Source: CAD feature listing. Evaluate the final solid. Frame: model axes, mm. A direction names the side the tool comes from. Give positions to 0.01 mm unless a question says otherwise; leave off trailing zeros. Write each loop counter-clockwise with the first axis right and the second up, starting at its lowest first coordinate (ties: lowest second). Pieces come first, ordered by that corner, then holes.
```python
from build123d import *

# Parameters (mm, degrees)
F1_DEPTH      = 50.8
F3_DEPTH      = 49.1127015481
F3_DEPTH_BACK = 66.494050136
F4_R          = 5.0698297576
F4_W          = 24.7860401869
F4_H          = 10.0980177522
F5_DEPTH      = 86.2099544535
F5_DEPTH_BACK = 86.2099544535


with BuildPart() as f1:
    # F0 (on Top) → F1 (new body)
    with BuildSketch(Plane.XY):
        Polygon((-86.2089544535, 49.1117015481), (-86.2089544535, -49.1117015481), (-12.8575693816, -49.1117015481), (-12.8575693816, -66.493050136), (9.0635353699, -66.493050136), (9.0635353699, -49.1117015481), (86.2089544535, -49.1117015481), (86.2089544535, 49.1117015481), align=None)
    extrude(amount=F1_DEPTH)

    # F2 (on Front) → F3 (cut, two sides)
    with BuildSketch(Plane.XZ) as f3_sk:
        Polygon((9.0635353699, 50.8), (-12.8575693816, 50.8), (86.2089544535, 0), (86.2089544535, 50.8), align=None)
    extrude(amount=-F3_DEPTH, mode=Mode.SUBTRACT)
    extrude(f3_sk.sketch, amount=F3_DEPTH_BACK, mode=Mode.SUBTRACT)

    # F4 (on Right) → F5 (cut, two sides)
    with BuildSketch(Plane.YZ) as f5_sk:
        with Locations((-29.1465427727, 37.8675609827)):
            Circle(F4_R)
        with Locations((-29.1465427727, 14.9175236002)):
            Circle(F4_R)
        with Locations((20.425543189, 14.9175236002)):
            Circle(F4_R)
        with Locations((20.425543189, 37.8675609827)):
            Circle(F4_R)
        with Locations((-8.0325044692, 45.7509911239)):
            Rectangle(F4_W, F4_H)
    extrude(amount=-F5_DEPTH, mode=Mode.SUBTRACT)
    extrude(f5_sk.sketch, amount=F5_DEPTH_BACK, mode=Mode.SUBTRACT)


solid = f1.part
```
1. Access query for faces 5 (the cylindrical face through (-8.53, 19.327, 9.968)), 6 (the flat face through (-12.858, -58, 25)), 7 (the flat face through (39, -49.112, 15)), 8 (the flat face through (-39, -20.426, 46)), 9 (the flat face through (-50, -35, 50.8)). Directions: +Z, -Z, +X, -X, +Y, -Y. A direction counts if a zero-diameter tool reaches every point of the face in a straight line with its end or side. Return the directions, or none.
2. Cut plane C-C, the plane y = -9. Return the cut outline in (x, z), then the cut area to 3 significant figures.
3. Cut plane B-B, the plane x = -16. Return the cut outline in (y, z), then the cut area to 3 significant figures.
4. Contact query for flat-ended pins moving along their axis: P1, Ø3, axis at x = -52, z = 45, coming from the -Y side; P2, Ø8.5, axis at y = -55, z = 33, coming from the -X side; P3, Ø4, axis at x = 61.5, z = 14, coming from the +Y side; P4, Ø12.5, axis at x = -38.5, y = -12.5, coming from the +Z side. Output: stop coordinate, or through.
5. Mould query, pull axis Y, two halves, no side actions, for faces 1 (the flat face through (35.982, -9.5, 25.756)), 2 (the cylindrical face through (-8.53, -26.81, 10.42)), 3 (the flat face through (-39, -8, 40.702)), 4 (the flat face through (-50, -49.112, 25)). Classes: +Y half, -Y half, draft (parallel to the pull), parting line (faces both ways), or undercut.
6. Line query: L1, parallel to Y at x = -78.5, z = 38.5; L2, parallel to Y at x = -31, z = 39.5; L3, parallel to Z at x = -41.5, y = 2. Output: solid intervals per line, ascending.
7. Cut plane D-D, the plane z = 22. Return the cut outline in (x, y), then the cut area to 3 significant figures.
8. Cut plane A-A, the plane z = 13. Return the cut outline in (x, y), then the cut area to 3 significant figures.
Response values:
1. face 5: +X, -X
1. face 6: +Z, -Z, -X, -Y
1. face 7: +Z, -Z, +X, -Y
1. face 8: +Z, +X, -X
1. face 9: +Z, +X, -X, +Y, -Y
2. outline: (-86.21, 0) - (86.21, 0) - (6.83, 40.7) - (-86.21, 40.7) - close
2. area: 5,400 mm2
3. outline: (-49.11, 0) - (49.11, 0) - (49.11, 50.8) - (4.36, 50.8) - (4.36, 40.7) - (-20.43, 40.7) - (-20.43, 50.8) - (-49.11, 50.8) - close; hole circle Ø10.14 at (-29.15, 14.92); hole circle Ø10.14 at (-29.15, 37.87); hole circle Ø10.14 at (20.43, 14.92); hole circle Ø10.14 at (20.43, 37.87)
3. area: 4,420 mm2
4. P1: stops at y = -49.11
4. P2: stops at x = -12.86
4. P3: stops at y = 49.11
4. P4: stops at z = 40.7
5. face 1: draft
5. face 2: undercut
5. face 3: undercut
5. face 4: -Y half
6. L1: y = -49.11 to -34.18, -24.12 to 15.4, 25.46 to 49.11
6. L2: y = -49.11 to -33.95, -24.35 to 15.63, 25.23 to 49.11
6. L3: z = 0 to 40.7
7. outline: (-86.21, -49.11) - (-12.86, -49.11) - (-12.86, -66.49) - (9.06, -66.49) - (9.06, -49.11) - (43.31, -49.11) - (43.31, 49.11) - (-86.21, 49.11) - close
7. area: 13,100 mm2
8. outline: (-86.21, -49.11) - (-12.86, -49.11) - (-12.86, -66.49) - (9.06, -66.49) - (9.06, -49.11) - (60.86, -49.11) - (60.86, -33.84) - (-86.21, -33.84) - close; (-86.21, -24.45) - (60.86, -24.45) - (60.86, 15.73) - (-86.21, 15.73) - close; (-86.21, 25.12) - (60.86, 25.12) - (60.86, 49.11) - (-86.21, 49.11) - close
8. area: 12,100 mm2
